Design review of the part built by this model. Coordinates are the model's own, in mm. A direction names the side the tool comes from. Give positions to 0.01 mm unless a question says otherwise; leave off trailing zeros. Write each loop counter-clockwise with the first axis right and the second up, starting at its lowest first coordinate (ties: lowest second). Pieces come first, ordered by that corner, then holes. Notation, with made-up numbers: (-16.5, 40.5) -> (2.5, 40.5) arc R24 cw to (2.5, 54.5) -> close; hole circle Ø10 at (29, 63.5). An arc over 180 degrees is marked (long way). Use CSV: the item, a comma, the result in double quotes.
```python
from build123d import *

# Parameters (mm, degrees)
SKETCH1_W               = 37.5
SKETCH1_H               = 7
BOSS_EXTRUDE1_DEPTH     = 10
CUT_EXTRUDE1_DEPTH      = 40.436658073
CUT_EXTRUDE1_DEPTH_BACK = 40.436658073
SKETCH2_R               = 3.75
FILLET1_R               = 2.54
F_4_0MM_DOWEL_HOLE1_D   = 4.75
CUT_EXTRUDE2_DEPTH      = 40.436658073
CUT_EXTRUDE2_DEPTH_BACK = 40.436658073
CUT_EXTRUDE3_DEPTH      = 3.5
FILLET2_R               = 2.54


with BuildPart() as part:
    # Sketch1 → Boss-Extrude1 (new body)
    with BuildSketch(Plane.XY):
        with Locations((18.75, 3.5)):
            Rectangle(SKETCH1_W, SKETCH1_H)
    extrude(amount=BOSS_EXTRUDE1_DEPTH)

    # Sketch2 → Cut-Extrude1 (cut, two sides: drawn at the far end of the back side and taken through both)
    with BuildSketch(Plane.XY.offset(10).offset(-CUT_EXTRUDE1_DEPTH_BACK)):
        with Locations((18.75, 0)):
            Circle(SKETCH2_R)
    extrude(amount=CUT_EXTRUDE1_DEPTH + CUT_EXTRUDE1_DEPTH_BACK, mode=Mode.SUBTRACT)

    # Fillet1
    fillet1_edges = [part.edges().sort_by_distance(p)[0] for p in [
        (37.5, 3.5, 10),
        (0, 3.5, 10),
        (37.5, 3.5, 0),
        (0, 3.5, 0),
    ]]
    fillet(fillet1_edges, radius=FILLET1_R)

    # Ø4.0mm Dowel Hole1 (through all)
    with Locations(Plane(origin=(0, 7, 0), x_dir=(1, 0, 0), z_dir=(0, 1, 0))):
        with Locations((5, -5), (32.5, -5)):
            Hole(F_4_0MM_DOWEL_HOLE1_D / 2)

    # Sketch6 → Cut-Extrude2 (cut, two sides: drawn at the far end of the back side and taken through both)
    with BuildSketch(Plane(origin=(0, 0, 0), x_dir=(-1, 0, 0), z_dir=(0, 0, -1)).offset(-CUT_EXTRUDE2_DEPTH_BACK)):
        Polygon((-2.54, 0), (-18.100943668, 3.693403021), (-18.100943668, 0), align=None)
    extrude(amount=CUT_EXTRUDE2_DEPTH + CUT_EXTRUDE2_DEPTH_BACK, mode=Mode.SUBTRACT)

    # Sketch7 → Cut-Extrude3 (cut)
    with BuildSketch(Plane.XZ):
        with BuildLine():
            Line((22.5, 6.78008281), (22.5, 0))
            Line((22.5, 0), (30.734125825, 0))
            ThreePointArc((30.734125825, 0), (25.400966559, 1.913143457), (22.5, 6.78008281))
        make_face()
        with BuildLine():
            Line((22.5, 10), (20.085032716, 10))
            Line((20.085032716, 10), (20.085032716, 0))
            Line((20.085032716, 0), (22.5, 0))
            Line((22.5, 0), (22.5, 6.78008281))
            ThreePointArc((22.5, 6.78008281), (22.34408442, 8.390041405), (22.5, 10))
        make_face()
    extrude(amount=-CUT_EXTRUDE3_DEPTH, mode=Mode.SUBTRACT)

    # Fillet2
    # the kernel refuses this fillet: 2.54 mm, written as the material it takes off along each edge
    with BuildSketch(Plane(origin=(16.15, 0, 10), x_dir=(0, 1, 0), z_dir=(1, 0, 0))) as fillet2_piece_1:
        with BuildLine():
            CenterArc((FILLET2_R, -FILLET2_R), FILLET2_R, 90, 90)
            Line((0, -FILLET2_R), (0, 0))
            Line((0, 0), (FILLET2_R, 0))
        make_face()
    extrude(amount=18.81, mode=Mode.SUBTRACT)
    with BuildSketch(Plane(origin=(34.96, 0, 7.46), x_dir=(0, 0, 1), z_dir=(-1, 0, 0))) as fillet2_piece_2:
        with BuildLine():
            CenterArc((2.54 - FILLET2_R, FILLET2_R), FILLET2_R, 270, 90)
            Line((2.54 - FILLET2_R, 0), (2.54, 0))
            Line((2.54, 0), (2.54, FILLET2_R))
        make_face()
    revolve(axis=Axis((34.96, 0, 7.46), (0, 1, 0)), revolution_arc=90, mode=Mode.SUBTRACT)
    with BuildSketch(Plane(origin=(37.5, 0, 2.54), x_dir=(-1, 0, 0), z_dir=(0, 0, 1))) as fillet2_piece_3:
        with BuildLine():
            CenterArc((FILLET2_R, -FILLET2_R), FILLET2_R, 90, 90)
            Line((0, -FILLET2_R), (0, 0))
            Line((0, 0), (FILLET2_R, 0))
        make_face()
    extrude(amount=4.92, mode=Mode.SUBTRACT)
    with BuildSketch(Plane(origin=(34.96, 0, 2.54), x_dir=(0, 0, -1), z_dir=(-1, 0, 0))) as fillet2_piece_4:
        with BuildLine():
            CenterArc((2.54 - FILLET2_R, -FILLET2_R), FILLET2_R, 0, 90)
            Line((2.54, -FILLET2_R), (2.54, 0))
            Line((2.54, 0), (2.54 - FILLET2_R, 0))
        make_face()
    revolve(axis=Axis((34.96, 0, 2.54), (0, -1, 0)), revolution_arc=90, mode=Mode.SUBTRACT)
    with BuildSketch(Plane(origin=(30.734125825, 0, 0), x_dir=(0, 1, 0), z_dir=(1, 0, 0))) as fillet2_piece_5:
        with BuildLine():
            CenterArc((FILLET2_R, FILLET2_R), FILLET2_R, 180, 90)
            Line((0, FILLET2_R), (0, 0))
            Line((0, 0), (FILLET2_R, 0))
        make_face()
    extrude(amount=4.225874175, mode=Mode.SUBTRACT)
    with BuildSketch(Plane(origin=(30.734125825, 0, 8.390041405), x_dir=(-0.8451253375205291, 0, 0.5345682032077963), z_dir=(0.5345682032077963, 0, 0.8451253375205291))) as fillet2_piece_6:
        with BuildLine():
            CenterArc((8.390041405 - FILLET2_R, -FILLET2_R), FILLET2_R, 0, 90)
            Line((8.390041405, -FILLET2_R), (8.390041405, 0))
            Line((8.390041405, 0), (8.390041405 - FILLET2_R, 0))
        make_face()
    revolve(axis=Axis((30.734125825, 0, 8.390041405), (0, -1, 0)), revolution_arc=122.314632757, mode=Mode.SUBTRACT)


solid = part.part
```
(1) Clearance check with flat-ended pins moving along their axes: pin 1 (4 mm diameter, centred on x = 14, z = 7, fed in from -Y); pin 2 (6 mm diameter, centred on x = 5, z = 5, fed in from -Y); pin 3 (4 mm diameter, centred on x = 32.5, z = 5, fed in from +Y); pin 4 (1 mm diameter, centred on x = 22, z = 1, fed in from -Y). State where each tip first meets the part, or that it passes through.
Established:
pin 1,"stops at y = 2.25"
pin 2,"stops at y = 0"
pin 3,"passes through"
pin 4,"stops at y = 3.5"
(2) Take a section at D-D (x = 22). Write out the cut boundary in (y, z), then the cut area to 3 significant figures.
Established:
outline,"(3.5, 0) -> (7, 0) -> (7, 10) -> (3.5, 10) -> close"
area,"35.0 mm2"
(3) Take a section at A-A (x = 32.5). Write out the cut boundary in (y, z) (3 decimals), then the cut area to 3 significant figures.
Established:
outline,"(0, 2.54) arc R2.54 ccw to (2.54, 0) -> (7, 0) -> (7, 2.625) -> (0, 2.625) -> close; (0, 7.375) -> (7, 7.375) -> (7, 10) -> (2.54, 10) arc R2.54 ccw to (0, 7.46) -> close"
area,"34.0 mm2"
(4) For line 1 along X through (y, z) = (5, 6); line 2 along Z through (x, y) = (5, 5) (3 decimals); line 3 along X through (y, z) = (4.75, 3.25), list the stretches that pass through material, from the lowest coordinate up. Write a range as [from, to].
Established:
line 1,"x = [0, 2.85], [7.15, 30.35], [34.65, 37.5]"
line 2,"z = [0, 2.625], [7.375, 10]"
line 3,"x = [0, 3.39], [6.61, 30.89], [34.11, 37.5]"
(5) Take a section at C-C (z = 3). State how many separate pieces and enclosed holes the cut face has, then the cut area to 3 significant figures.
Established:
separate pieces,"3"
enclosed holes,"0"
area,"174 mm2"
(6) Tool access review of faces 4 (the face through (32.817, 0.724, 0.764)), 5 (the face through (28.643, 0.764, 9.276)), 6 (the face through (10, 1.77, 5.07)): name each direction out of +Z, -Z, +X, -X, +Y, -Y from which nothing blocks a thin tool from reaching the whole face with its end or side.
Established:
face 4,"-Z, +X, -Y"
face 5,"+Z, +X, -Y"
face 6,"+Z, -Z, -Y"
(7) Take a section at B-B (x = 5). Write out the cut boundary in (y, z) (3 decimals).
Established:
outline,"(0.584, 0) -> (7, 0) -> (7, 2.625) -> (0.584, 2.625) -> close; (0.584, 7.375) -> (7, 7.375) -> (7, 10) -> (0.584, 10) -> close"
(8) Mouldability with a two-part tool opening along X and no side actions: class faces 1 (the face through (34.38, 3.45, 6.45)), 2 (the face through (29, 0, 6)), 3 (the face through (0.724, 3.549, 0.764)) as +X half, -X half, draft (parallel to the pull), parting line (faces both ways), or undercut.
Established:
face 1,"undercut"
face 2,"draft"
face 3,"-X half"
